Build history of the part. All positions in model axes, mm. Face numbers are marked on the shaded views. A direction names the side the tool comes from. Round coordinates to 2 decimals unless told otherwise and drop trailing zeros. Loops run counter-clockwise (first coordinate to the right, second up) from the corner with the lowest first, then second, coordinate; pieces in that order, holes last.
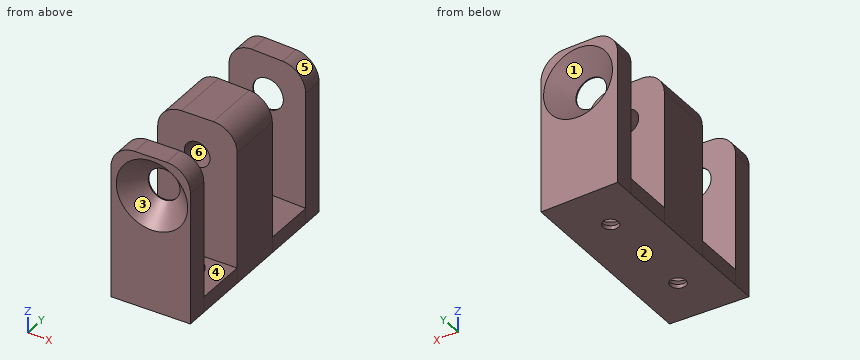
Autodesk Inventor part; units mm, degrees
ref_plane "YZ Plane" through (0, 0, 0) normal (1, 0, 0) x (0, 1, 0)
ref_plane "XZ Plane" through (0, 0, 0) normal (0, 1, 0) x (-1, 0, 0)
ref_plane "XY Plane" through (0, 0, 0) normal (0, 0, 1) x (1, 0, 0)
sketch "Skizze1" plane through (0, 0, 0) normal (0, 0, 1) x (1, 0, 0)
  line L0 (12.8939, 29.9442) -> (2.8939, 30.2214)
  line L1 (2.8939, 30.2214) -> (2.8939, 27.5773)
  line L2 (2.8939, 27.5773) -> (12.8939, 27.3001)
  line L3 (12.8939, 27.3001) -> (12.8939, 29.9442)
  line L4 (12.8939, 7.1427) -> (2.8939, 6.8655)
  line L5 (2.8939, 6.8655) -> (2.8939, 4.2214)
  line L6 (2.8939, 4.2214) -> (12.8939, 4.4985)
  line L7 (12.8939, 4.4985) -> (12.8939, 7.1427)
  line L8 (2.8939, 20.9747) -> (12.8939, 20.6975)
  line L9 (12.8939, 13.7452) -> (2.8939, 13.468)
  line L10 (16.8904, 10.5547) -> (7.8939, 10.3054) construction
  line L11 (16.8904, 23.888) -> (7.8939, 24.1374) construction
  line L12 (16.8904, 10.5547) -> (16.8904, 23.888) construction
  line L13 (2.8939, 20.9747) -> (12.8939, 27.3001) construction
  line L14 (2.8939, 13.468) -> (12.8939, 7.1427) construction
  line L15 (2.8939, 13.468) -> (2.8939, 20.9747)
  line L16 (12.8939, 13.7452) -> (12.8939, 20.6975)
  point P0 (7.8939, 7.0041)
  dimension "d36" = 9
  dimension "d37" = 13.3333
  dimension "d38" = 91.588
  dimension "d39" = 91.588
  dimension "d40" = 10
  dimension "d41" = 6.6
  dimension "d42" = 6.6
  dimension "d43" = 13.8321
  dimension "d58" = 26
extrude "Extrusion1" add sketch "Skizze1" along normal blind 20
fillet "Rundung1" radius 3 6 edges at (12.8939, 5.8206, 20) (12.8939, 28.6221, 20) (2.8939, 28.8993, 20) (2.8939, 5.5434, 20) (12.8939, 17.2214, 20) (2.8939, 17.2214, 20)
sketch "Skizze4" plane through (2.8939, 22.0416, 0) normal (0, 0, 1) x (1, 0, 0)
  line L0 (9.5, -17.8202) -> (0.5, -17.8202) construction
  line L1 (7, 7.9858) -> (3, 8.0966) construction
  line L2 (5, -11.7363) -> (5, -11.4869) construction
  line L3 (5, 1.8464) -> (5, 2.0958) construction
  dimension "d59" = 13.3333
sketch "Skizze6" plane through (2.8939, 4.2214, 0) normal (0, 0, -1) x (0.9992829, 0.0378646, 0)
  line L0 (10.9668, -25.3257) -> (0.9845, -25.9814)
  line L1 (0, 0) -> (10.0033, 0.1017)
  line L2 (0.9845, -25.9814) -> (0, 0)
  line L3 (10.9668, -25.3257) -> (10.0033, 0.1017)
extrude "Extrusion3" add sketch "Skizze6" against normal blind 2
hole "Bohrung4" at (7.8939, 10.5547, 0) at (7.8939, 23.888, 0) direction (0, 0, 1) diameter 2 end through all
chamfer "Fasen1" distance 1.5 angle 45 2 edges at (7.8939, 22.888, 2) (7.8939, 9.5547, 2)
sketch "Skizze7" plane through (12.8939, 4.4985, 0) normal (0.0277065, -0.9996161, 0) x (0.9996161, 0.0277065, 0)
  line L0 (-4.8372, 0) -> (-4.8372, 15) construction
  point P0 (-13.0135, 0)
  dimension "d60" = 15
hole "Bohrung5" at (8.0585, 4.3645, 15) direction (-0.0277065, 0.9996161, 0) diameter 4 depth 2.6431 countersink diameter 9 countersink angle 90
sketch "Skizze8" plane through (12.8939, 4.4985, 0) normal (0.0277065, -0.9996161, 0) x (0.9996161, 0.0277065, 0)
  circle A0 centre (-4.7839, 15) radius 2.0011
  point P0 (-13.0135, 0)
hole "Bohrung6" at (8.1118, 4.366, 15) direction (-0.0277065, 0.9996161, 0) diameter 3.242 depth 13 tip angle 118
sketch "Skizze9" plane through (2.8939, 30.2214, 17) normal (0.0277065, 0.9996161, 0) x (0.9996161, -0.0277065, 0)
  line L0 (5.1666, 17) -> (5.1666, 2) construction
  point P0 (-2.0554, 17)
  dimension "d75" = 15
hole "Bohrung7" at (8.0585, 30.0782, 15) direction (-0.0277065, -0.9996161, 0) diameter 4 depth 2.6431 countersink diameter 9 countersink angle 90
sketch "Skizze10" plane through (2.8939, 30.2214, 17) normal (0.0277065, 0.9996161, 0) x (0.9996161, -0.0277065, 0)
  circle A0 centre (5.2233, 2) radius 2.0011
  point P0 (-2.0554, 17)
hole "Bohrung8" at (8.1152, 30.0767, 15) direction (-0.0277065, -0.9996161, 0) diameter 3.242 depth 13 tip angle 118
properties part number "HalterUmlenkrolleDPL" material "PC/ABS-Kunststoff, 3DDruck, PLA"
(1) Slice it at B-B on y = 26.75. List the corners of the cut face in (x, z), plus the area to 3 significant figures.
Responses:
outline: (2.89, 0) - (12.89, 0) - (12.89, 2) - (2.89, 2) - close
area: 20.0 mm2
(2) Pin check, flat tips, straight feed: P1, Ø12, axis at y = 27, z = 5.5, coming from the +X side; P2, Ø1.5, axis at x = 6.5, z = 8.5, coming from the +Y side; P3, Ø6, axis at x = 10.5, z = 6.5, coming from the -Y side. Stop position of each tip, or through.
Responses:
P1: stops at x = 12.89
P2: stops at y = 30.14
P3: stops at y = 4.35
(3) Pull direction Y, two halves, no side cores. Call the marked faces 1, 2, 3 and 4: +Y half, -Y half, draft (parallel to the pull), parting line (faces both ways), or undercut.
Responses:
face 1: +Y half
face 2: draft
face 3: -Y half
face 4: undercut
(4) Which spindle directions (+Z, -Z, +X, -X, +Y, -Y) get a long thin tool onto all of the face, cutting with end or side? Do the marked faces 5 and 6. Say none if no direction does.
Responses:
face 5: +Z, +X, +Y, -Y
face 6: none
(5) Slice it at C-C on z = 16.25. Count the separate pieces of the cut face and the enclosed holes in it, plus the area to 3 significant figures.
Responses:
separate pieces: 6
enclosed holes: 0
area: 79.5 mm2
(6) Probe line 1 (Y direction, x = 4.75, z = 12.5); line 2 (Y direction, x = 9, z = 11.5); line 3 (Z direction, x = 11, y = 24.5). List the from-to ranges inside material, lowest first.
Responses:
line 1: y = 4.63 to 6.92, 13.52 to 20.92, 27.53 to 29.81
line 2: y = 5.26 to 7.03, 13.64 to 20.81, 27.41 to 29.18
line 3: z = 0 to 2
(7) Slice it at A-A on z = 5.25. List the corners of the cut face in (x, y).
Responses:
outline: (2.89, 4.22) - (12.89, 4.5) - (12.89, 7.14) - (2.89, 6.87) - close; (2.89, 13.47) - (12.89, 13.75) - (12.89, 20.7) - (2.89, 20.97) - close; (2.89, 27.58) - (12.89, 27.3) - (12.89, 29.94) - (2.89, 30.22) - close
